```python
from build123d import *

# Parameters (mm, degrees)
VERRUNDUNG1_R = 1.2
FASE1_SIZE    = 0.5


with BuildPart() as part:
    # Skizze1 → Rotation1 (revolve)
    with BuildSketch(Plane(origin=(0, 0, 0), x_dir=(0, 0, -1), z_dir=(1, 0, 0))):
        Polygon((0, 2.7), (0, 1.5), (8, 1.5), (8, 0), (-2.1, 0), (-2.1, 2.7), align=None)
    revolve(axis=Axis((0, 0, 0), (0, 0, -1)))

    # Verrundung1
    verrundung1_edges = [part.edges().sort_by_distance(p)[0] for p in [
        (0, -2.7, 2.1),
    ]]
    fillet(verrundung1_edges, radius=VERRUNDUNG1_R)

    # Fase1
    fase1_edges = [part.edges().sort_by_distance(p)[0] for p in [
        (0, -1.5, -8),
    ]]
    chamfer(fase1_edges, length=FASE1_SIZE)


solid = part.part
```
Model file for the job. Use its own axes, mm. A direction names the side the tool comes from. Round coordinates to 2 decimals unless told otherwise and drop trailing zeros. Write each loop counter-clockwise with the first axis right and the second up, starting at its lowest first coordinate (ties: lowest second). Pieces come first, ordered by that corner, then holes. Notation, with made-up numbers: (58, 15.25) - (68, 15.25) arc R28 ccw to (68, 54.25) - close; hole circle Ø2 at (53.25, 0). An arc over 180 degrees is marked (long way). One line per item, written item: value.
(1) Cut at D-D, the plane z = 0.75. Give the cut face in (x, y).
Values follow:
outline: circle Ø5.4 at (0, 0)
(2) 3-axis set-ups, long thin cutter, end or side, ignore diameter. For faces 1 (the cylindrical face through (-2.636, -0.585, 0.444)), 2 (the flat face through (-1.2, 1.2, 0)): which of +Z, -Z, +X, -X, +Y, -Y reach the whole face in a straight line?
Values follow:
face 1: +Z, -Z
face 2: -Z
(3) Drop flat-ended pins along their axis: P1, Ø1.6, axis at x = -1, y = 1, coming from the -Z side; P2, Ø2, axis at x = 1, y = -2, coming from the -Z side. Give the stop position or say it passes through.
Values follow:
P1: stops at z = -8
P2: stops at z = -7.76
(4) Cut at A-A, the plane x = 0. Give the cut face in (y, z).
Values follow:
outline: (-2.7, 0) - (-1.5, 0) - (-1.5, -7.5) - (-1, -8) - (1, -8) - (1.5, -7.5) - (1.5, 0) - (2.7, 0) - (2.7, 0.9) arc R1.2 ccw to (1.5, 2.1) - (-1.5, 2.1) arc R1.2 ccw to (-2.7, 0.9) - close
(5) Wall check: probe 1 along Z at (x, y) = (1.45, 0.5); probe 2 along Y at (x, z) = (1.3, -6.25); probe 3 along Y at (x, z) = (1.95, 1.5). Give the ranges that are in metal, low to high.
Values follow:
probe 1: z = 0 to 2.1
probe 2: y = -0.75 to 0.75
probe 3: y = -1.63 to 1.63
(6) Cut at C-C, the plane z = -2.75. Give the cut face in (x, y).
Values follow:
outline: circle Ø3 at (0, 0)
